from build123d import *

# Parameters (mm, degrees)
SKETCH1_W           = 279.4
SKETCH1_H           = 38.1
BOSS_EXTRUDE1_DEPTH = 9.525
SKETCH2_W           = 12.7
SKETCH2_H           = 9.525
BOSS_EXTRUDE2_DEPTH = 9.525
SKETCH3_R           = 2.3368
CUT_EXTRUDE1_DEPTH  = 10.525


with BuildPart() as part:
    # Sketch1 → Boss-Extrude1 (new body)
    with BuildSketch(Plane(origin=(0, 0, 0), x_dir=(1, 0, 0), z_dir=(0, 1, 0))):
        Rectangle(SKETCH1_W, SKETCH1_H)
    extrude(amount=BOSS_EXTRUDE1_DEPTH)

    # Sketch2 → Boss-Extrude2 (add)
    with BuildSketch(Plane(origin=(139.7, 0, 0), x_dir=(0, 0, -1), z_dir=(1, 0, 0))):
        with Locations((0, 4.7625)):
            Rectangle(SKETCH2_W, SKETCH2_H)
    boss_extrude2 = extrude(amount=BOSS_EXTRUDE2_DEPTH)

    # Mirror1: Boss-Extrude2 across plane
    add(boss_extrude2.mirror(Plane(origin=(0, 0, 0), x_dir=(0, 0, 1), z_dir=(1, 0, 0))))

    # Sketch3 → Cut-Extrude1 (cut, through all)
    with BuildSketch(Plane.XZ):
        with Locations((114.3, -8.7376)):
            Circle(SKETCH3_R)
        with Locations((77.7748, -8.7376)):
            Circle(SKETCH3_R)
        with Locations((96.0374, -8.7376)):
            Circle(SKETCH3_R)
    cut_extrude1 = extrude(amount=-CUT_EXTRUDE1_DEPTH, mode=Mode.SUBTRACT)

    # Mirror2: Cut-Extrude1 across plane
    add(cut_extrude1.mirror(Plane(origin=(0, 0, 0), x_dir=(0, 0, 1), z_dir=(1, 0, 0))), mode=Mode.SUBTRACT)


solid = part.part
For this review, take the finished solid that the model builds, in its own axes (mm). A direction names the side the tool comes from. Round coordinates to 2 decimals unless told otherwise and drop trailing zeros. Order: outer loops, then holes, each group sorted by start corner. A loop starts at its lowest first (then second) coordinate and runs counter-clockwise, first axis right, second up. Notation, with made-up numbers: M 3,45 L 20,45 A25 cw 20,59 Z; hole C 39.25,45 d1. An arc over 180 degrees is marked long. Use a Markdown table: item, result. Add a question column.
Item 1: Add section A-A, the plane z = -16. Give the boundary of the cut face in (x, y) (3 decimals), then the cut area to 3 significant figures.
Item 2: To check wall thickness, follow line 1 along Z through (x, y) = (-114.3, 3.25); line 2 along X through (y, z) = (5, -16.5); line 3 along Z through (x, y) = (-95.5, 2.25). State the ranges of each line that lie inside material, in increasing order.
Item 3: Insertion check: pin 1 (5 mm diameter, centred on y = 6, z = -14.5, fed in from +X); pin 2 (4 mm diameter, centred on x = 114.3, z = -8.74, fed in from -Y) (3 decimals); pin 3 (1.5 mm diameter, centred on y = 6.5, z = 10.5, fed in from -X); pin 4 (5 mm diameter, centred on x = 145, y = 6.5, fed in from +Z). Each pin has a flat end and moves straight along its axis. Give the tip position at first contact, or say it passes through.
Item 4: Tool access review of faces 1 (the flat face through (-144, 5, -6.35)), 2 (the flat face through (144, 5, -6.35)), 3 (the flat face through (139.7, 5, 13)), 4 (the flat face through (-139.7, 5, 13)), 5 (the flat face through (-2, 5, -19.05)): name each direction out of +Z, -Z, +X, -X, +Y, -Y from which nothing blocks a thin tool from reaching the whole face with its end or side.
Item 5: Add section B-B, the plane y = 4.25. Give the boundary of the cut face in (x, z) (3 decimals), then the cut area to 3 significant figures.
Item 6: Mouldability with a two-part tool opening along Z and no side actions: class faces 6 (the flat face through (-144, 5, 6.35)), 7 (the flat face through (139.7, 5, -13)), 8 (the cylindrical face through (93.703, 4.696, -8.635)), 9 (the cylindrical face through (-75.44, 4.7, -8.63)) as released by +Z, released by -Z, zero draft, split by the parting line, or undercut.
Geometry results:
| question | item | result |
|---|---|---|
| 1 | outline | M -139.7,0 L 139.7,0 L 139.7,9.525 L -139.7,9.525 Z |
| 1 | area | 2,660 mm² |
| 2 | line 1 | z = -19.05 to -11.07, -6.4 to 19.05 |
| 2 | line 2 | x = -139.7 to 139.7 |
| 2 | line 3 | z = -19.05 to -11.01, -6.46 to 19.05 |
| 3 | pin 1 | stops at x = 139.7 |
| 3 | pin 2 | passes through |
| 3 | pin 3 | stops at x = -139.7 |
| 3 | pin 4 | stops at z = 6.35 |
| 4 | face 1 | -Z, -X, +Y, -Y |
| 4 | face 2 | -Z, +X, +Y, -Y |
| 4 | face 3 | +Z, +X, +Y, -Y |
| 4 | face 4 | +Z, -X, +Y, -Y |
| 4 | face 5 | -Z, +X, -X, +Y, -Y |
| 5 | outline | M -149.225,-6.35 L -139.7,-6.35 L -139.7,-19.05 L 139.7,-19.05 L 139.7,-6.35 L 149.225,-6.35 L 149.225,6.35 L 139.7,6.35 L 139.7,19.05 L -139.7,19.05 L -139.7,6.35 L -149.225,6.35 Z; hole C -114.3,-8.738 d4.674; hole C -96.037,-8.738 d4.674; hole C -77.775,-8.738 d4.674; hole C 77.775,-8.738 d4.674; hole C 96.037,-8.738 d4.674; hole C 114.3,-8.738 d4.674 |
| 5 | area | 10,800 mm² |
| 6 | face 6 | released by +Z |
| 6 | face 7 | zero draft |
| 6 | face 8 | undercut |
| 6 | face 9 | undercut |
